```python
from build123d import *

# Parameters (mm, degrees)
BOSS_EXTRUDE1_DEPTH = 3
SKETCH2_R           = 1.35
CUT_EXTRUDE1_DEPTH  = 4
SKETCH4_R           = 1.35
CUT_EXTRUDE2_DEPTH  = 4
SKETCH5_R           = 1.35
CUT_EXTRUDE3_DEPTH  = 4
SKETCH6_R           = 1.35
CUT_EXTRUDE4_DEPTH  = 4
FILLET1_R           = 3
SKETCH7_R           = 1.75
CUT_EXTRUDE5_DEPTH  = 4
LPATTERN1_COUNT     = 2
LPATTERN1_PITCH     = 24
SKETCH8_R           = 1.35
CUT_EXTRUDE6_DEPTH  = 4
SKETCH9_R           = 1.5
CUT_EXTRUDE7_DEPTH  = 4
CUT_EXTRUDE8_DEPTH  = 4
FILLET2_R           = 1
FILLET3_R           = 4
SKETCH11_W          = 17
SKETCH11_H          = 6.5
CUT_EXTRUDE9_DEPTH  = 4


with BuildPart() as part:
    # Sketch1 → Boss-Extrude1 (new body)
    with BuildSketch(Plane(origin=(0, 0, 0), x_dir=(1, 0, 0), z_dir=(0, 1, 0))):
        Polygon((0, 27.8), (0, -27.8), (32, -27.8), (32, -40.3), (156, -40.3), (156, -27.3), (111, -27.3), (111, 27.3), (156, 27.3), (156, 40.3), (32, 40.3), (32, 27.8), align=None)
    extrude(amount=BOSS_EXTRUDE1_DEPTH)

    # Sketch2 → Cut-Extrude1 (cut, through all)
    with BuildSketch(Plane(origin=(0, 3, 0), x_dir=(1, 0, 0), z_dir=(0, 1, 0))):
        with Locations((3, 8.7)):
            Circle(SKETCH2_R)
        with Locations((3, 24.9)):
            Circle(SKETCH2_R)
        with Locations((3, -8.7)):
            Circle(SKETCH2_R)
        with Locations((3, -24.9)):
            Circle(SKETCH2_R)
    cut_extrude1 = extrude(amount=-CUT_EXTRUDE1_DEPTH, mode=Mode.SUBTRACT)

    # Sketch4 → Cut-Extrude2 (cut, through all)
    with BuildSketch(Plane(origin=(0, 3, 0), x_dir=(1, 0, 0), z_dir=(0, 1, 0))):
        with Locations((75, -36.3)):
            Circle(SKETCH4_R)
        with Locations((75, 36.3)):
            Circle(SKETCH4_R)
    extrude(amount=-CUT_EXTRUDE2_DEPTH, mode=Mode.SUBTRACT)

    # Sketch5 → Cut-Extrude3 (cut, through all)
    with BuildSketch(Plane(origin=(0, 3, 0), x_dir=(1, 0, 0), z_dir=(0, 1, 0))):
        with Locations((103, 22)):
            Circle(SKETCH5_R)
        with Locations((103, -22)):
            Circle(SKETCH5_R)
    extrude(amount=-CUT_EXTRUDE3_DEPTH, mode=Mode.SUBTRACT)

    # Sketch6 → Cut-Extrude4 (cut, through all)
    with BuildSketch(Plane(origin=(0, 3, 0), x_dir=(1, 0, 0), z_dir=(0, 1, 0))):
        with Locations((120, 31.3)):
            Circle(SKETCH6_R)
        with Locations((152, 31.3)):
            Circle(SKETCH6_R)
        with Locations((120, -31.3)):
            Circle(SKETCH6_R)
        with Locations((152, -31.3)):
            Circle(SKETCH6_R)
    extrude(amount=-CUT_EXTRUDE4_DEPTH, mode=Mode.SUBTRACT)

    # Fillet1
    fillet1_edges = [part.edges().sort_by_distance(p)[0] for p in [
        (111, 1.5, 27.3),
        (111, 1.5, -27.3),
    ]]
    fillet(fillet1_edges, radius=FILLET1_R)

    # Sketch7 → Cut-Extrude5 (cut, through all)
    with BuildSketch(Plane(origin=(0, 3, 0), x_dir=(1, 0, 0), z_dir=(0, 1, 0))):
        with Locations((101.5, 0)):
            Circle(SKETCH7_R)
        with Locations((87.210580838, 8.25)):
            Circle(SKETCH7_R)
        with Locations((87.210580838, -8.25)):
            Circle(SKETCH7_R)
    extrude(amount=-CUT_EXTRUDE5_DEPTH, mode=Mode.SUBTRACT)

    # LPattern1: Cut-Extrude1 ×2
    with Locations(*[(i * LPATTERN1_PITCH, 0, 0) for i in range(1, LPATTERN1_COUNT)]):
        add(cut_extrude1, mode=Mode.SUBTRACT)

    # Sketch8 → Cut-Extrude6 (cut, through all)
    with BuildSketch(Plane(origin=(0, 3, 0), x_dir=(1, 0, 0), z_dir=(0, 1, 0))):
        with Locations((3, 18.5)):
            Circle(SKETCH8_R)
        with Locations((27, 18.5)):
            Circle(SKETCH8_R)
        with Locations((3, -18.5)):
            Circle(SKETCH8_R)
        with Locations((27, -18.5)):
            Circle(SKETCH8_R)
        with Locations((3, 0)):
            Circle(SKETCH8_R)
        with Locations((27, 0)):
            Circle(SKETCH8_R)
    extrude(amount=-CUT_EXTRUDE6_DEPTH, mode=Mode.SUBTRACT)

    # Sketch9 → Cut-Extrude7 (cut, through all)
    with BuildSketch(Plane(origin=(0, 3, 0), x_dir=(1, 0, 0), z_dir=(0, 1, 0))):
        with Locations((65.8, 22.6)):
            Circle(SKETCH9_R)
        with Locations((64.53, -25.66)):
            Circle(SKETCH9_R)
    extrude(amount=-CUT_EXTRUDE7_DEPTH, mode=Mode.SUBTRACT)

    # Sketch10 → Cut-Extrude8 (cut, through all)
    with BuildSketch(Plane(origin=(0, 3, 0), x_dir=(1, 0, 0), z_dir=(0, 1, 0))):
        Polygon((37, 5), (61.5, 5), (61.5, 25), (42, 25), (37, 20), align=None)
        Polygon((37, -5), (61.5, -5), (61.5, -25), (42, -25), (37, -20), align=None)
    extrude(amount=-CUT_EXTRUDE8_DEPTH, mode=Mode.SUBTRACT)

    # Fillet2
    fillet2_edges = [part.edges().sort_by_distance(p)[0] for p in [
        (0, 1.5, -27.8),
        (0, 1.5, 27.8),
        (32, 1.5, 40.3),
        (156, 1.5, 40.3),
        (156, 1.5, 27.3),
        (156, 1.5, -27.3),
        (156, 1.5, -40.3),
        (32, 1.5, -40.3),
    ]]
    fillet(fillet2_edges, radius=FILLET2_R)

    # Fillet3
    fillet3_edges = [part.edges().sort_by_distance(p)[0] for p in [
        (32, 1.5, 27.8),
        (32, 1.5, -27.8),
    ]]
    fillet(fillet3_edges, radius=FILLET3_R)

    # Sketch11 → Cut-Extrude9 (cut, through all)
    with BuildSketch(Plane(origin=(0, 3, 0), x_dir=(1, 0, 0), z_dir=(0, 1, 0))):
        with Locations((89.5, 29)):
            Rectangle(SKETCH11_W, SKETCH11_H)
        with Locations((89.5, -32)):
            Rectangle(SKETCH11_W, SKETCH11_H)
    extrude(amount=-CUT_EXTRUDE9_DEPTH, mode=Mode.SUBTRACT)


solid = part.part
```
Can you work these out from the model? Positions are in its coordinate system, mm. A direction names the side the tool comes from. Give positions to 0.01 mm unless a question says otherwise; leave off trailing zeros. Loops run counter-clockwise (first coordinate to the right, second up) from the corner with the lowest first, then second, coordinate; pieces in that order, holes last. Notation, with made-up numbers: M 76,-18.75 L 114,-18.75 A16 cw 114,-3.75 Z; hole C 25.5,-17.5 d3. An arc over 180 degrees is marked long. One line per question, with ' | ' between items. Start each with the question number.
Q1. If we section it at A-A (x = 132): Please give me the cut outline in (y, z), plus the area to 3 significant figures.
Q2. If we mould it in two halves opening along Z, with no side actions, what happens to faces 1 (the flat face through (32, 1, 35)), 2 (the cylindrical face through (30.859, 1.521, -29.003)), 3 (the cylindrical face through (3.62, 1.52, 26.1))? For each: +Z half, -Z half, draft (parallel to the pull), parting line (faces both ways), or undercut.
Q3. If we section it at C-C (x = 93.5): Please give me the cut outline in (y, z), plus the area to 3 significant figures.
Q4. If we section it at B-B (z = 15): Please give me the cut outline in (x, y), plus the area to 4 significant figures.
Q5. If I drill on line 1 (Z direction, x = 75, y = 2.9); line 2 (X direction, y = 1.9, z = 18.5); line 3 (Z direction, x = 92, y = 1.8), over which ranges is the centre line in solid material (lowest first)? Write a range as from..to.
Q6. If we section it at D-D (y = 1.8): State how many separate pieces and enclosed holes the cut face has, plus the area to 3 significant figures.
Q7. For faces 4 (the flat face through (15, 1, -27.8)), 5 (the flat face through (111, 1, 0)), 6 (the flat face through (89, 2, 35.25)), which set-ups out of +Z, -Z, +X, -X, +Y, -Y let a thin tool reach every point of the face, with its end or its side?
Q8. For pin 1 Ø0.9 at (x, y) = (13, 1) entering from +Z; pin 2 Ø2 at (x, z) = (152, -31.3) entering from +Y, each with a flat end and sliding along its axis, tell me the tip position at first contact or that it passes through.
Computed:
1) outline: M 0,-40.3 L 3,-40.3 L 3,-27.3 L 0,-27.3 Z; M 0,27.3 L 3,27.3 L 3,40.3 L 0,40.3 Z | area: 78.0 mm²
2) face 1: draft | face 2: -Z half | face 3: undercut
3) outline: M 0,-40.3 L 3,-40.3 L 3,-32.25 L 0,-32.25 Z; M 0,-25.75 L 3,-25.75 L 3,28.75 L 0,28.75 Z; M 0,35.25 L 3,35.25 L 3,40.3 L 0,40.3 Z | area: 203 mm²
4) outline: M 0,0 L 37,0 L 37,3 L 0,3 Z; M 61.5,0 L 111,0 L 111,3 L 61.5,3 Z | area: 259.5 mm²
5) line 1: z = -40.3..-37.65, -34.95..34.95, 37.65..40.3 | line 2: x = 0..1.65, 4.35..25.65, 28.35..37, 61.5..111 | line 3: z = -40.3..-32.25, -25.75..28.75, 35.25..40.3
6) separate pieces: 1 | enclosed holes: 31 | area: 7,980 mm²
7) face 4: -Z, -X, +Y, -Y | face 5: +X, +Y, -Y | face 6: +Y, -Y
8) pin 1: stops at z = 27.8 | pin 2: passes through
